Verification items for this drawing (mm, ordinates from the low corner). Give positions to 0.01 mm unless a question says otherwise; leave off trailing zeros. Order: outer loops, then holes, each group sorted by start corner. A loop starts at its lowest first (then second) coordinate and runs counter-clockwise, first axis right, second up. Notation, with made-up numbers: M 85,-28 L 116,-28 A19 cw 116,9 Z; hole C -18,23 d9. An arc over 180 degrees is marked long. Answer as a JSON object with one key per item and string values.
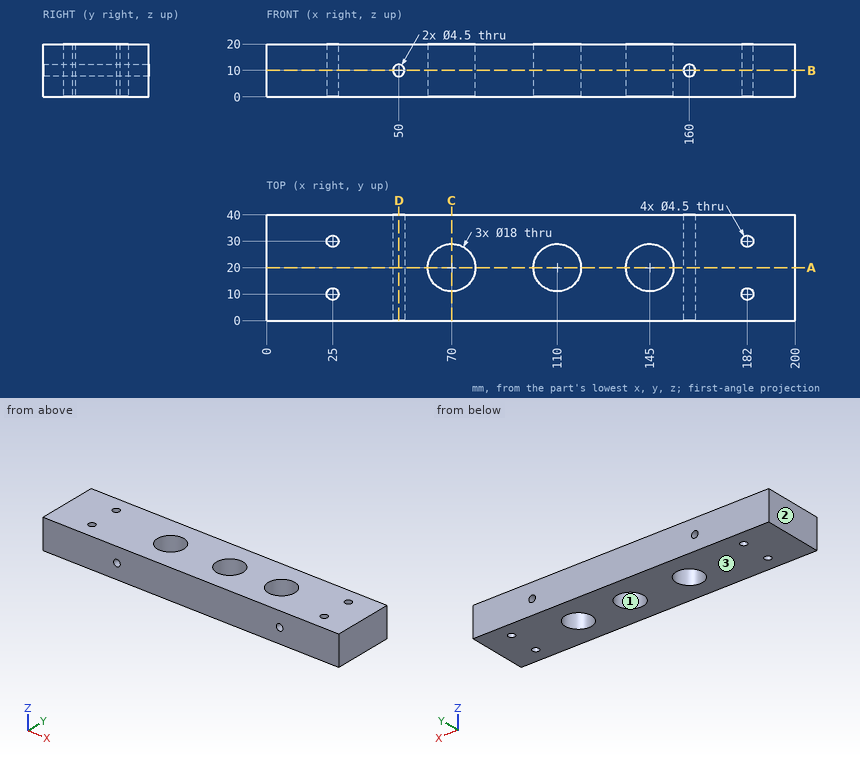
Q1. Section check D-D on x = 50. Record the cut outline in (y, z).
Resolved:
{"outline": "M 0,0 L 40,0 L 40,7.75 L 0,7.75 Z; M 0,12.25 L 40,12.25 L 40,20 L 0,20 Z"}
Q2. Section check C-C on x = 70. Record the cut outline in (y, z).
Resolved:
{"outline": "M 0,0 L 11,0 L 11,20 L 0,20 Z; M 29,0 L 40,0 L 40,20 L 29,20 Z"}
Q3. Section check B-B on z = 10. Count the separate pieces of the cut face and the enclosed holes in it, then the cut area to 3 significant figures.
Resolved:
{"separate pieces": "3", "enclosed holes": "7", "area": "6,810 mm²"}
Q4. Gauge pin test, flat end, axial feed: pin 1 Ø2.5 at (x, y) = (182, 10) entering from +Z. Record the tip position at first contact, or that the pin passes through.
Resolved:
{"pin 1": "passes through"}
Q5. Material ranges on L1, parallel to Y at x = 182, z = 14; L2, parallel to X at y = 10, z = 7.5; L3, parallel to Y at x = 145, z = 4, recorded low to high.
Resolved:
{"L1": "y = 0 to 7.75, 12.25 to 27.75, 32.25 to 40", "L2": "x = 0 to 22.75, 27.25 to 179.75, 184.25 to 200", "L3": "y = 0 to 11, 29 to 40"}
Q6. Section check A-A on y = 20. Record the cut outline in (x, z), then the cut area to 3 significant figures.
Resolved:
{"outline": "M 0,0 L 61,0 L 61,20 L 0,20 Z; M 79,0 L 101,0 L 101,20 L 79,20 Z; M 119,0 L 136,0 L 136,20 L 119,20 Z; M 154,0 L 200,0 L 200,20 L 154,20 Z; hole C 50,10 d4.5; hole C 160,10 d4.5", "area": "2,890 mm²"}
Q7. Release check for a two-part mould opening along X. For the marked faces 1, 2 and 3 record: +X half, -X half, draft (parallel to the pull), parting line (faces both ways), or undercut.
Resolved:
{"face 1": "undercut", "face 2": "-X half", "face 3": "draft"}
